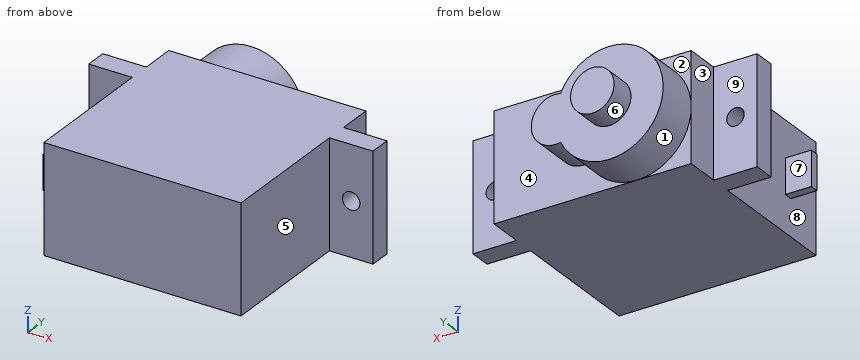
```python
from build123d import *

# Parameters (mm, degrees)
SALIENTE_EXTRUIR1_DEPTH = 12.4
SALIENTE_EXTRUIR2_DEPTH = 5
CROQUIS3_R              = 2.5
SALIENTE_EXTRUIR3_DEPTH = 3
CROQUIS4_W              = 4
CROQUIS4_H              = 1
SALIENTE_EXTRUIR4_DEPTH = 3
CROQUIS5_R              = 1
CORTAR_EXTRUIR1_DEPTH   = 2.5


with BuildPart() as part:
    # Croquis1 → Saliente-Extruir1 (new body)
    with BuildSketch(Plane.XY):
        Polygon((-22.65, 18.25), (-22.65, 22.25), (0, 22.25), (0, 18.25), (5, 18.25), (5, 15.75), (0, 15.75), (0, 0), (-22.65, 0), (-22.65, 15.75), (-27.65, 15.75), (-27.65, 18.25), align=None)
    extrude(amount=SALIENTE_EXTRUIR1_DEPTH)

    # Croquis2 → Saliente-Extruir2 (add)
    with BuildSketch(Plane(origin=(0, 22.25, 0), x_dir=(1, 0, 0), z_dir=(0, 1, 0))):
        with BuildLine():
            ThreePointArc((-10.859879032, -3.518480363), (-22.65, -6.2), (-10.859879032, -8.881519637))
            ThreePointArc((-10.859879032, -8.881519637), (-7.5, -6.2), (-10.859879032, -3.518480363))
        make_face()
    extrude(amount=SALIENTE_EXTRUIR2_DEPTH)

    # Croquis3 → Saliente-Extruir3 (add)
    with BuildSketch(Plane(origin=(0, 27.25, 0), x_dir=(1, 0, 0), z_dir=(0, 1, 0))):
        with Locations(Location((-16.45, -6.2, 0), (0, 0, 180))):
            Circle(CROQUIS3_R)
    extrude(amount=SALIENTE_EXTRUIR3_DEPTH)

    # Croquis4 → Saliente-Extruir4 (add)
    with BuildSketch(Plane.ZY.offset(22.65)):
        with Locations((6.2, 5)):
            Rectangle(CROQUIS4_W, CROQUIS4_H)
    extrude(amount=SALIENTE_EXTRUIR4_DEPTH)

    # Croquis5 → Cortar-Extruir1 (cut)
    with BuildSketch(Plane(origin=(0, 18.25, 0), x_dir=(1, 0, 0), z_dir=(0, 1, 0))):
        with Locations(Location((2.5, -6.2, 0), (0, 0, 270))):
            Circle(CROQUIS5_R)
        with Locations(Location((-25.15, -6.2, 0), (0, 0, 270))):
            Circle(CROQUIS5_R)
    extrude(amount=-CORTAR_EXTRUIR1_DEPTH, mode=Mode.SUBTRACT)


solid = part.part
```
Can you work these out from the model? Positions are in its coordinate system, mm. Face numbers are marked on the shaded views. A direction names the side the tool comes from. Give positions to 0.01 mm unless a question says otherwise; leave off trailing zeros. Loops run counter-clockwise (first coordinate to the right, second up) from the corner with the lowest first, then second, coordinate; pieces in that order, holes last. Notation, with made-up numbers: M -16,12 L 32,12 A13 ccw 32,21 Z; hole C -30.5,-4.75 d3. An arc over 180 degrees is marked long. Answer in a Markdown table with one row per item.
1. Suppose I cut it at C-C on z = 5.75. Count the separate pieces of the cut face and the enclosed holes in it, plus the area to 3 significant figures.
Taken from the geometry:
| item | result |
|---|---|
| separate pieces | 3 |
| enclosed holes | 0 |
| area | 613 mm² |
2. Suppose I cut it at D-D on x = -25.15. Write out the boundary of the cut face in (y, z), plus the area to 3 significant figures.
Taken from the geometry:
| item | result |
|---|---|
| outline | M 4.5,4.2 L 5.5,4.2 L 5.5,8.2 L 4.5,8.2 Z; M 15.75,0 L 18.25,0 L 18.25,5.2 L 15.75,5.2 Z; M 15.75,7.2 L 18.25,7.2 L 18.25,12.4 L 15.75,12.4 Z |
| area | 30.0 mm² |
3. Suppose I cut it at B-B on x = -10.25. Write out the boundary of the cut face in (y, z), plus the area to 3 significant figures.
Taken from the geometry:
| item | result |
|---|---|
| outline | M 0,0 L 22.25,0 L 22.25,3.45 L 27.25,3.45 L 27.25,8.95 L 22.25,8.95 L 22.25,12.4 L 0,12.4 Z |
| area | 303 mm² |
4. Which directions (+Z, -Z, +X, -X, +Y, -Y) give clear straight access to the entire face, cutting with the end or side of a thin tool? Please do the marked faces 1, 2, 3, 4 and 5.
Taken from the geometry:
| item | result |
|---|---|
| face 1 | +Y |
| face 2 | +Z, -X, +Y |
| face 3 | +Z, -Z, -X, +Y |
| face 4 | +X, +Y |
| face 5 | +Z, -Z, +X, -Y |
5. Suppose I cut it at A-A on x = 2.5. Write out the boundary of the cut face in (y, z), plus the area to 3 significant figures.
Taken from the geometry:
| item | result |
|---|---|
| outline | M 15.75,0 L 18.25,0 L 18.25,5.2 L 15.75,5.2 Z; M 15.75,7.2 L 18.25,7.2 L 18.25,12.4 L 15.75,12.4 Z |
| area | 26.0 mm² |
6. For pin 1 Ø1.5 at (x, z) = (-24, 6.5) entering from +Y; pin 2 Ø1.6 at (x, z) = (2.5, 6.2) entering from +Y; pin 3 Ø1.5 at (x, z) = (-24.5, 5.5) entering from -Y; pin 4 Ø6 at (y, z) = (7.5, 5) entering from -X, each with a flat end and sliding along its axis, tell me the tip position at first contact or that it passes through.
Taken from the geometry:
| item | result |
|---|---|
| pin 1 | stops at y = 18.25 |
| pin 2 | passes through |
| pin 3 | stops at y = 4.5 |
| pin 4 | stops at x = -25.65 |
7. If I drill on line 1 along X through (y, z) = (16.5, 6.2); line 2 along Y through (x, z) = (-13, 11.25); line 3 along X through (y, z) = (10, 5), over which ranges is the centre line in solid material (lowest first)?
Taken from the geometry:
| item | result |
|---|---|
| line 1 | x = -27.65 to -26.15, -24.15 to 1.5, 3.5 to 5 |
| line 2 | y = 0 to 27.25 |
| line 3 | x = -22.65 to 0 |
8. Thinking about a two-plate mould opening in Y: for the marked faces 6, 7, 8 and 9, which applies, released by +Y, released by -Y, zero draft, split by the parting line, or undercut?
Taken from the geometry:
| item | result |
|---|---|
| face 6 | zero draft |
| face 7 | undercut |
| face 8 | undercut |
| face 9 | released by +Y |
